```python
from build123d import *

# Parameters (mm, degrees)
SKETCH1_R           = 15
SKETCH1_R_2         = 12.5
BOSS_EXTRUDE1_DEPTH = 17
BOSS_EXTRUDE2_START = -6
SKETCH1_3_R         = 20.913430936
SKETCH1_3_R_2       = 15.913430936
SKETCH1_3_R_3       = 15
SKETCH1_3_R_4       = 12.5
BOSS_EXTRUDE2_DEPTH = 6
CUT_EXTRUDE1_START  = -4
SKETCH1_4_R         = 20.913430936
SKETCH1_4_R_2       = 15.913430936
CUT_EXTRUDE1_DEPTH  = 2


with BuildPart() as part:
    # Sketch1 → Boss-Extrude1 (new body)
    with BuildSketch(Plane(origin=(0, 0, 0), x_dir=(1, 0, 0), z_dir=(0, 1, 0))):
        with Locations(Location((0, 0, 0), (0, 0, 270))):
            Circle(SKETCH1_R)
        with Locations(Location((0, 0, 0), (0, 0, 270))):
            Circle(SKETCH1_R_2, mode=Mode.SUBTRACT)
    extrude(amount=BOSS_EXTRUDE1_DEPTH)

    # Sketch1_3 → Boss-Extrude2 (add)
    # profile 1 of 3: a face of its own
    with BuildSketch(Plane(origin=(0, 0, 0), x_dir=(1, 0, 0), z_dir=(0, 1, 0)).offset(BOSS_EXTRUDE2_START)):
        with Locations(Location((0, 0, 0), (0, 0, 270))):
            Circle(SKETCH1_3_R)
        Circle(SKETCH1_3_R_2, mode=Mode.SUBTRACT)
    # profile 2 of 3: a face of its own
    with BuildSketch(Plane(origin=(0, 0, 0), x_dir=(1, 0, 0), z_dir=(0, 1, 0)).offset(BOSS_EXTRUDE2_START)):
        Circle(SKETCH1_3_R_2)
        with Locations(Location((0, 0, 0), (0, 0, 270))):
            Circle(SKETCH1_3_R_3, mode=Mode.SUBTRACT)
    # profile 3 of 3: a face of its own
    with BuildSketch(Plane(origin=(0, 0, 0), x_dir=(1, 0, 0), z_dir=(0, 1, 0)).offset(BOSS_EXTRUDE2_START)):
        with Locations(Location((0, 0, 0), (0, 0, 270))):
            Circle(SKETCH1_3_R_3)
        with Locations(Location((0, 0, 0), (0, 0, 270))):
            Circle(SKETCH1_3_R_4, mode=Mode.SUBTRACT)
    extrude(amount=BOSS_EXTRUDE2_DEPTH)

    # Sketch1_4 → Cut-Extrude1 (cut)
    with BuildSketch(Plane(origin=(0, 0, 0), x_dir=(1, 0, 0), z_dir=(0, 1, 0)).offset(CUT_EXTRUDE1_START)):
        with Locations(Location((0, 0, 0), (0, 0, 270))):
            Circle(SKETCH1_4_R)
        with Locations(Location((0, 0, 0), (0, 0, 270))):
            Circle(SKETCH1_4_R_2, mode=Mode.SUBTRACT)
    extrude(amount=CUT_EXTRUDE1_DEPTH, mode=Mode.SUBTRACT)


solid = part.part
```
Verification items for the finished model (mm, model axes). A direction names the side the tool comes from. Give positions to 0.01 mm unless a question says otherwise; leave off trailing zeros. Loops run counter-clockwise (first coordinate to the right, second up) from the corner with the lowest first, then second, coordinate; pieces in that order, holes last.
1. Mould release check, pull along Y, two halves, no side actions. Record for faces 4 (the flat face through (-14, 0, 9)), 5 (the flat face through (-15.4, -2, -4.7)), 6 (the cylindrical face through (3.755, 5.339, 11.923)), 7 (the flat face through (-9, -6, 9)): released by +Y, released by -Y, zero draft, split by the parting line, or undercut.
2. Section check A-A, the plane x = 0. Enter the section's corners in (y, z).
3. Go/stop test with flat-tipped pins: pin 1 Ø4 at (x, y) = (11.5, 11.5) entering from -Z; pin 2 Ø6 at (x, y) = (13, -0.5) entering from +Z; pin 3 Ø5 at (x, y) = (-13.5, 12.5) entering from +Z. Record where each tip stops, or that it passes through.
4. Thickness scan on line 1 (Y direction, x = -15.5, z = -9.5); line 2 (X direction, y = 8, z = 0); line 3 (X direction, y = -0.5, z = 0). Record the ranges inside material, lowest first.
5. Section check B-B, the plane z = 0. Enter the section's corners in (x, y), then the cut area to 3 significant figures.
6. Section check C-C, the plane x = 14. Enter the section's corners in (y, z).
7. Set-up check for faces 1 (the flat face through (-15.4, -4, -4.7)), 2 (the cylindrical face through (0.66, 8.381, -14.985)), 3 (the flat face through (12.3, 17, -3.4)): record each of +Z, -Z, +X, -X, +Y, -Y from which the full face is reachable in a straight line by a thin tool's end or side.
8. Section check D-D, the plane y = 8. Enter the section's corners in (x, z).
Geometry says:
1. face 4: released by +Y
1. face 5: undercut
1. face 6: zero draft
1. face 7: released by -Y
2. outline: (-6, -20.91) - (-4, -20.91) - (-4, -15.91) - (-2, -15.91) - (-2, -20.91) - (0, -20.91) - (0, -15) - (17, -15) - (17, -12.5) - (-6, -12.5) - close; (-6, 12.5) - (17, 12.5) - (17, 15) - (0, 15) - (0, 20.91) - (-2, 20.91) - (-2, 15.91) - (-4, 15.91) - (-4, 20.91) - (-6, 20.91) - close
3. pin 1: stops at z = -11.61
3. pin 2: stops at z = 18.37
3. pin 3: stops at z = 10.2
4. line 1: y = -6 to -4, -2 to 0
4. line 2: x = -15 to -12.5, 12.5 to 15
4. line 3: x = -20.91 to -12.5, 12.5 to 20.91
5. outline: (-20.91, -6) - (-12.5, -6) - (-12.5, 17) - (-15, 17) - (-15, 0) - (-20.91, 0) - (-20.91, -2) - (-15.91, -2) - (-15.91, -4) - (-20.91, -4) - close; (12.5, -6) - (20.91, -6) - (20.91, -4) - (15.91, -4) - (15.91, -2) - (20.91, -2) - (20.91, 0) - (15, 0) - (15, 17) - (12.5, 17) - close
5. area: 166 mm2
6. outline: (-6, -15.54) - (-4, -15.54) - (-4, -7.57) - (-2, -7.57) - (-2, -15.54) - (0, -15.54) - (0, -5.39) - (17, -5.39) - (17, 5.39) - (0, 5.39) - (0, 15.54) - (-2, 15.54) - (-2, 7.57) - (-4, 7.57) - (-4, 15.54) - (-6, 15.54) - close
7. face 1: none
7. face 2: +Y
7. face 3: +Z, -Z, +X, -X, +Y
8. outline: circle Ø30 at (0, 0); hole circle Ø25 at (0, 0)
